```python
from build123d import *

# Parameters (mm, degrees)
F1_DEPTH = 5
F2_R     = 22.5
F3_DEPTH = 7
F5_DEPTH = 12.5


with BuildPart() as f1:
    # F0 (on Front) → F1 (new body, symmetric)
    with BuildSketch(Plane.XZ):
        with BuildLine():
            Line((6.5, 73), (6.5, 38.5))
            ThreePointArc((6.5, 38.5), (4.5961940777, 33.9038059223), (0, 32))
            ThreePointArc((0, 32), (-4.5961940777, 33.9038059223), (-6.5, 38.5))
            Line((-6.5, 38.5), (-6.5, 73))
            ThreePointArc((-6.5, 73), (-9.566281029, 72.6617937246), (-12.6156130875, 72.1948495838))
            ThreePointArc((-12.6156130875, 72.1948495838), (-28.294097646, 49.0068146771), (-56.2147672182, 47.02286621))
            ThreePointArc((-56.2147672182, 47.02286621), (-58.1438187355, 44.6155392532), (-59.9698544763, 42.1291651246))
            Line((-59.9698544763, 42.1291651246), (-30.0919780457, 24.8791651246))
            ThreePointArc((-30.0919780457, 24.8791651246), (-27.0634601748, 20.9323237932), (-27.7128129211, 16))
            ThreePointArc((-27.7128129211, 16), (-31.6596542525, 12.9714821291), (-36.5919780457, 13.6208348754))
            Line((-36.5919780457, 13.6208348754), (-66.4698544763, 30.8708348754))
            ThreePointArc((-66.4698544763, 30.8708348754), (-67.7100997645, 28.0462544714), (-68.8303803057, 25.1719833738))
            ThreePointArc((-68.8303803057, 25.1719833738), (-56.5881952919, 0), (-68.8303803057, -25.1719833738))
            ThreePointArc((-68.8303803057, -25.1719833738), (-67.7100997645, -28.0462544714), (-66.4698544763, -30.8708348754))
            Line((-66.4698544763, -30.8708348754), (-36.5919780457, -13.6208348754))
            ThreePointArc((-36.5919780457, -13.6208348754), (-31.6596542525, -12.9714821291), (-27.7128129211, -16))
            ThreePointArc((-27.7128129211, -16), (-27.0634601748, -20.9323237932), (-30.0919780457, -24.8791651246))
            Line((-30.0919780457, -24.8791651246), (-59.9698544763, -42.1291651246))
            ThreePointArc((-59.9698544763, -42.1291651246), (-58.1438187355, -44.6155392532), (-56.2147672182, -47.02286621))
            ThreePointArc((-56.2147672182, -47.02286621), (-28.294097646, -49.0068146771), (-12.6156130875, -72.1948495838))
            ThreePointArc((-12.6156130875, -72.1948495838), (-9.566281029, -72.6617937246), (-6.5, -73))
            Line((-6.5, -73), (-6.5, -38.5))
            ThreePointArc((-6.5, -38.5), (-4.5961940777, -33.9038059223), (0, -32))
            ThreePointArc((0, -32), (4.5961940777, -33.9038059223), (6.5, -38.5))
            Line((6.5, -38.5), (6.5, -73))
            ThreePointArc((6.5, -73), (9.566281029, -72.6617937246), (12.6156130875, -72.1948495838))
            ThreePointArc((12.6156130875, -72.1948495838), (28.294097646, -49.0068146771), (56.2147672182, -47.02286621))
            ThreePointArc((56.2147672182, -47.02286621), (58.1438187355, -44.6155392532), (59.9698544763, -42.1291651246))
            Line((59.9698544763, -42.1291651246), (30.0919780457, -24.8791651246))
            ThreePointArc((30.0919780457, -24.8791651246), (27.0634601748, -20.9323237932), (27.7128129211, -16))
            ThreePointArc((27.7128129211, -16), (31.6596542525, -12.9714821291), (36.5919780457, -13.6208348754))
            Line((36.5919780457, -13.6208348754), (66.4698544763, -30.8708348754))
            ThreePointArc((66.4698544763, -30.8708348754), (67.7100997645, -28.0462544714), (68.8303803057, -25.1719833738))
            ThreePointArc((68.8303803057, -25.1719833738), (56.5881952919, 0), (68.8303803057, 25.1719833738))
            ThreePointArc((68.8303803057, 25.1719833738), (67.7100997645, 28.0462544714), (66.4698544763, 30.8708348754))
            Line((66.4698544763, 30.8708348754), (36.5919780457, 13.6208348754))
            ThreePointArc((36.5919780457, 13.6208348754), (31.6596542525, 12.9714821291), (27.7128129211, 16))
            ThreePointArc((27.7128129211, 16), (27.0634601748, 20.9323237932), (30.0919780457, 24.8791651246))
            Line((30.0919780457, 24.8791651246), (59.9698544763, 42.1291651246))
            ThreePointArc((59.9698544763, 42.1291651246), (58.1438187355, 44.6155392532), (56.2147672182, 47.02286621))
            ThreePointArc((56.2147672182, 47.02286621), (28.294097646, 49.0068146771), (12.6156130875, 72.1948495838))
            ThreePointArc((12.6156130875, 72.1948495838), (9.566281029, 72.6617937246), (6.5, 73))
        make_face()
    extrude(amount=F1_DEPTH, both=True)

    # F2 (on Front) → F3 (join, symmetric)
    with BuildSketch(Plane.XZ):
        Circle(F2_R)
    extrude(amount=F3_DEPTH, both=True)

    # F4 (on Front) → F5 (cut, symmetric)
    with BuildSketch(Plane.XZ):
        with BuildLine():
            ThreePointArc((-3.25, 12.2771128528), (-7.7464508002, -10.0639207072), (12.7, 0))
            ThreePointArc((12.7, 0), (10.0639207072, 7.7464508002), (3.25, 12.2771128528))
            Line((3.25, 12.2771128528), (-3.25, 12.2771128528))
        make_face()
        with BuildLine():
            Line((-3.25, 12.2771128528), (3.25, 12.2771128528))
            ThreePointArc((3.25, 12.2771128528), (0, 12.7), (-3.25, 12.2771128528))
        make_face()
        with BuildLine():
            ThreePointArc((-3.25, 12.2771128528), (0, 12.7), (3.25, 12.2771128528))
            Line((3.25, 12.2771128528), (3.25, 15.5271128528))
            Line((3.25, 15.5271128528), (-3.25, 15.5271128528))
            Line((-3.25, 15.5271128528), (-3.25, 12.2771128528))
        make_face()
    extrude(amount=F5_DEPTH, both=True, mode=Mode.SUBTRACT)


solid = f1.part
```
Part model, mm, in its own coordinate system. A direction names the side the tool comes from. Round coordinates to 2 decimals unless told otherwise and drop trailing zeros. Order: outer loops, then holes, each group sorted by start corner. A loop starts at its lowest first (then second) coordinate and runs counter-clockwise, first axis right, second up. Notation, with made-up numbers: M -7.5,14.5 L 17.5,14.5 A14 cw 17.5,19.5 Z; hole C 55,71 d5. An arc over 180 degrees is marked long. Answer in a Markdown table with one row per item. Add a question column.
Q1. Wall check: L1, parallel to Z at x = 31, y = 3; L2, parallel to Z at x = 39, y = -2.25; L3, parallel to X at y = 0, z = 0. Give the ranges that are in metal, low to high. Write a range as from..to.
Q2. Cut at A-A on x = 0. Give the cut face in (y, z).
Q3. Cut at C-C on x = 47.5. Give the cut face in (y, z).
Q4. Pin check, flat tips, straight feed: pin 1 (23 mm diameter, centred on x = 0, z = 0, fed in from -Y); pin 2 (6 mm diameter, centred on x = -19, y = -5, fed in from -Z); pin 3 (3 mm diameter, centred on x = 1, y = 1, fed in from -Z); pin 4 (5 mm diameter, centred on y = 2, z = -62.5, fed in from -X). Stop position of each tip, or through.
Q5. Cut at B-B on z = -19.25. Give the cut face in (x, y), and give its area (3 significant figures).
Q6. Cut at D-D on x = -14.5. Give the cut face in (y, z), and give its area (3 significant figures).
Q7. Mould opens along X. For faces 1 (the face through (-44.822, -0.07, -33.383)), 2 (the face through (-9.523, -0.07, 72.667)), 3 (the face through (-5.4, 5, 22)) say: +X half, -X half, draft (parallel to the pull), parting line (faces both ways), or undercut.
Q8. 3-axis set-ups, long thin cutter, end or side, ignore diameter. For faces 4 (the face through (6.5, 0, -56)), 5 (the face through (-51.322, -0.07, 22.125)), 6 (the face through (-5.4, -5, 22)): which of +Z, -Z, +X, -X, +Y, -Y reach the whole face in a straight line?
Established:
| question | item | result |
|---|---|---|
| 1 | L1 | z = -47.61..-25.4, -13.19..13.19, 25.4..47.61 |
| 1 | L2 | z = -45.16..-30.02, -15.01..15.01, 30.02..45.16 |
| 1 | L3 | x = -56.59..-12.7, 12.7..56.59 |
| 2 | outline | M -7,-22.5 L -5,-22.5 L -5,-32 L 5,-32 L 5,-22.5 L 7,-22.5 L 7,-12.7 L -7,-12.7 Z; M -7,15.53 L 7,15.53 L 7,22.5 L 5,22.5 L 5,32 L -5,32 L -5,22.5 L -7,22.5 Z |
| 3 | outline | M -5,-44.88 L 5,-44.88 L 5,-34.93 L -5,-34.93 Z; M -5,-19.92 L 5,-19.92 L 5,19.92 L -5,19.92 Z; M -5,34.93 L 5,34.93 L 5,44.88 L -5,44.88 Z |
| 4 | pin 1 | passes through |
| 4 | pin 2 | stops at z = -61.77 |
| 4 | pin 3 | stops at z = -32.5 |
| 4 | pin 4 | stops at x = -17.01 |
| 5 | outline | M -63.03,-5 L -46.34,-5 L -46.34,5 L -63.03,5 Z; M -26.84,-5 L -11.65,-5 L -11.65,-7 L 11.65,-7 L 11.65,-5 L 26.84,-5 L 26.84,5 L 11.65,5 L 11.65,7 L -11.65,7 L -11.65,5 L -26.84,5 Z; M 46.34,-5 L 63.03,-5 L 63.03,5 L 46.34,5 Z |
| 5 | area | 964 mm2 |
| 6 | outline | M -7,-17.2 L -5,-17.2 L -5,-65.04 L 5,-65.04 L 5,-17.2 L 7,-17.2 L 7,17.2 L 5,17.2 L 5,65.04 L -5,65.04 L -5,17.2 L -7,17.2 Z |
| 6 | area | 1,440 mm2 |
| 7 | face 1 | undercut |
| 7 | face 2 | -X half |
| 7 | face 3 | draft |
| 8 | face 4 | -Z, +Y, -Y |
| 8 | face 5 | +Y, -Y |
| 8 | face 6 | -Y |
